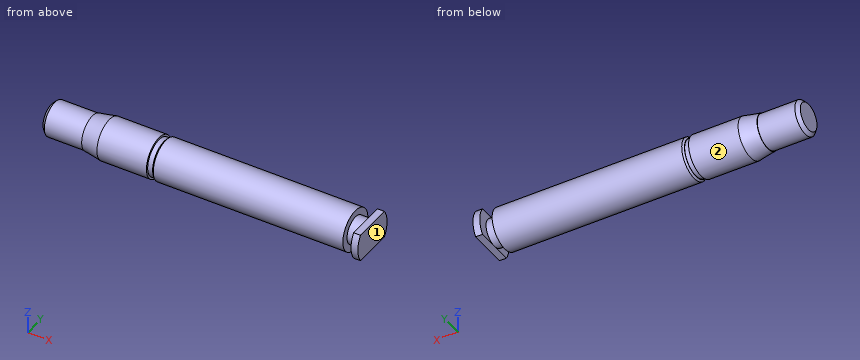
from build123d import *

# Parameters (mm, degrees)
CHANFREIN1_SIZE         = 1
CHANFREIN2_SIZE         = 0.5
ENL_V_MAT_EXTRU_1_REACH = 96.52
ESQUISSE2_W             = 5.137351374
ESQUISSE2_H             = 15.268552686


with BuildPart() as part:
    # Esquisse1 → Révolution1 (revolve)
    with BuildSketch(Plane.XY, mode=Mode.PRIVATE) as r_volution1_sk:
        Polygon((0, 0), (0, 5), (12, 5), (12, 5.118365096), (17, 6), (31.5, 6), (31.5, 5.4), (33, 5.4), (33, 6), (89, 6), (89, 4), (92, 4), (92, 7), (94, 7), (94, 0), align=None)
    revolve(r_volution1_sk.sketch.rotate(Axis((0, 0, 0), (1, 0, 0)), 90), axis=Axis((0, 0, 0), (1, 0, 0)))

    # Chanfrein1
    chanfrein1_edges = [part.edges().sort_by_distance(p)[0] for p in [
        (0, 0, -5),
    ]]
    chamfer(chanfrein1_edges, length=CHANFREIN1_SIZE)

    # Chanfrein2
    chanfrein2_edges = [part.edges().sort_by_distance(p)[0] for p in [
        (33, 0, -6),
    ]]
    chamfer(chanfrein2_edges, length=CHANFREIN2_SIZE)

    # Esquisse2 → Enlèv. mat.-Extru.1 (cut, up to next)
    with BuildSketch(Plane(origin=(94, 0, 0), x_dir=(0, 0, -1), z_dir=(1, 0, 0)), mode=Mode.PRIVATE) as enl_v_mat_extru_1_sk1:
        with Locations((-6.568675687, -0.086100861)):
            Rectangle(ESQUISSE2_W, ESQUISSE2_H)
    enl_v_mat_extru_1_tool1 = extrude(enl_v_mat_extru_1_sk1.sketch, amount=-ENL_V_MAT_EXTRU_1_REACH, mode=Mode.PRIVATE) & part.part
    # Esquisse2 → Enlèv. mat.-Extru.1 (cut, up to next)
    with BuildSketch(Plane(origin=(94, 0, 0), x_dir=(0, 0, -1), z_dir=(1, 0, 0)), mode=Mode.PRIVATE) as enl_v_mat_extru_1_sk2:
        with Locations((6.568675687, -0.086100861)):
            Rectangle(ESQUISSE2_W, ESQUISSE2_H)
    enl_v_mat_extru_1_tool2 = extrude(enl_v_mat_extru_1_sk2.sketch, amount=-ENL_V_MAT_EXTRU_1_REACH, mode=Mode.PRIVATE) & part.part
    add(enl_v_mat_extru_1_tool1.solids().sort_by_distance((94, -0.086101, 6.568676))[0], mode=Mode.SUBTRACT)
    add(enl_v_mat_extru_1_tool2.solids().sort_by_distance((94, -0.086101, -6.568676))[0], mode=Mode.SUBTRACT)


solid = part.part
Could you check a few things on this model? Use its own coordinates, in mm. Face numbers are marked on the shaded views. A direction names the side the tool comes from. Give positions to 0.01 mm unless a question says otherwise; leave off trailing zeros. Order: outer loops, then holes, each group sorted by start corner. A loop starts at its lowest first (then second) coordinate and runs counter-clockwise, first axis right, second up. Notation, with made-up numbers: (62.25, 63) - (101.25, 63) arc R29 ccw to (101.25, 85) - close; hole circle Ø9 at (62, 54.5). An arc over 180 degrees is marked (long way). One line per item, written item: value. Start each with the question number.
1. Imagine slicing it at B-B on x = 83. List the corners of the cut face in (y, z) for me.
2. For P1, Ø6, axis at x = 79, y = 4.5, coming from the +Z side; P2, Ø0.6, axis at x = 92.5, y = 1, coming from the -Z side; P3, Ø1, axis at x = 93, y = -1, coming from the +Z side, each with a flat end and sliding along its axis, tell me the tip position at first contact or that it passes through.
3. If I drill on probe 1 along X at (y, z) = (5, -3.5); probe 2 along X at (y, z) = (-3.25, -3.25); probe 3 along Z at (x, y) = (75.5, 0.25), over which ranges is the centre line in solid material (lowest first)?
4. For the marked faces 1 and 2, which set-ups out of +Z, -Z, +X, -X, +Y, -Y let a thin tool reach every point of the face, with its end or its side?
Values:
1. outline: circle Ø12 at (0, 0)
2. P1: z = 5.81
2. P2: z = -4
2. P3: z = 4
3. probe 1: 92 to 94
3. probe 2: 0.6 to 89, 92 to 94
3. probe 3: -5.99 to 5.99
4. face 1: +Z, -Z, +X, +Y, -Y
4. face 2: -X
